```python
from build123d import *

# Parameters (mm, degrees)
SKETCH1_W           = 20
SKETCH1_H           = 5
SKETCH1_R           = 1.5
BOSS_EXTRUDE1_DEPTH = 2


with BuildPart() as part:
    # Sketch1 → Boss-Extrude1 (new body)
    with BuildSketch(Plane(origin=(0, 0, 0), x_dir=(1, 0, 0), z_dir=(0, 1, 0))):
        Rectangle(SKETCH1_W, SKETCH1_H)
        with Locations(Location((-7.5, 0, 0), (0, 0, 270))):
            Circle(SKETCH1_R, mode=Mode.SUBTRACT)
        with Locations(Location((7.5, 0, 0), (0, 0, 270))):
            Circle(SKETCH1_R, mode=Mode.SUBTRACT)
        with Locations(Location((0, 0, 0), (0, 0, 270))):
            Circle(SKETCH1_R, mode=Mode.SUBTRACT)
    extrude(amount=BOSS_EXTRUDE1_DEPTH)


solid = part.part
```
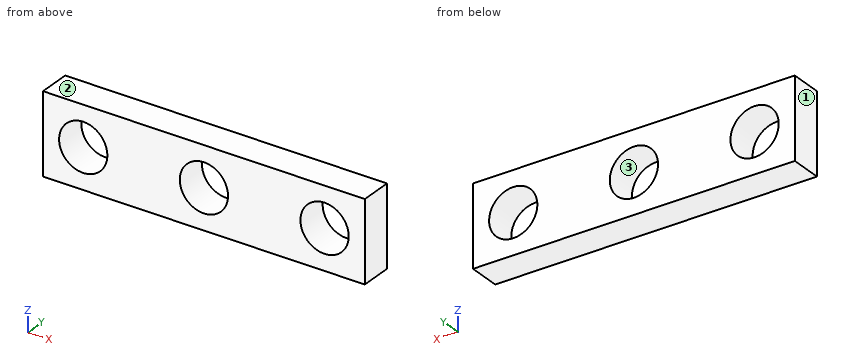
Check sheet for the modelled part. Datum: model origin and axes. Units: mm. Face numbers are marked on the shaded views. Give positions to 0.01 mm unless a question says otherwise; leave off trailing zeros. Write each loop counter-clockwise with the first axis right and the second up, starting at its lowest first coordinate (ties: lowest second). Pieces come first, ordered by that corner, then holes. Notation, with made-up numbers: (33.25, 57.5) -> (52.25, 57.5) arc R21 cw to (52.25, 78.5) -> close; hole circle Ø9 at (55, 42). An arc over 180 degrees is marked (long way). Use CSV: the item, a comma, the result in double quotes. Start each with the question number.
Q1. Scan lines: line 1 along X through (y, z) = (1.2, 0); line 2 along X through (y, z) = (0.6, 1.1); line 3 along Z through (x, y) = (1, 1.45). Record each from-to range of solid material in increasing order.
Q2. Release check for a two-part mould opening along Z. For the marked faces 1, 2 and 3 record: +Z half, -Z half, draft (parallel to the pull), parting line (faces both ways), or undercut.
Q3. Cross-section at D-D on z = -1.2. Enter the section's corners in (x, y).
Q4. Cross-section at B-B on z = 0. Enter the section's corners in (x, y), and give its area (3 significant figures).
Q5. Cross-section at A-A on x = 0. Enter the section's corners in (y, z).
Q6. Depth check by flat-ended pin: P1, Ø1.8, axis at x = 0, z = 0, coming from the -Y side. Enter the tip coordinate at first touch or a pass-through.
Q7. Cross-section at C-C on y = 0.35. Enter the section's corners in (x, z).
Working result:
1,line 1,"x = -10 to -9, -6 to -1.5, 1.5 to 6, 9 to 10"
1,line 2,"x = -10 to -8.52, -6.48 to -1.02, 1.02 to 6.48, 8.52 to 10"
1,line 3,"z = -2.5 to -1.12, 1.12 to 2.5"
2,face 1,"draft"
2,face 2,"+Z half"
2,face 3,"undercut"
3,outline,"(-10, 0) -> (-8.4, 0) -> (-8.4, 2) -> (-10, 2) -> close; (-6.6, 0) -> (-0.9, 0) -> (-0.9, 2) -> (-6.6, 2) -> close; (0.9, 0) -> (6.6, 0) -> (6.6, 2) -> (0.9, 2) -> close; (8.4, 0) -> (10, 0) -> (10, 2) -> (8.4, 2) -> close"
4,outline,"(-10, 0) -> (-9, 0) -> (-9, 2) -> (-10, 2) -> close; (-6, 0) -> (-1.5, 0) -> (-1.5, 2) -> (-6, 2) -> close; (1.5, 0) -> (6, 0) -> (6, 2) -> (1.5, 2) -> close; (9, 0) -> (10, 0) -> (10, 2) -> (9, 2) -> close"
4,area,"22.0 mm^2"
5,outline,"(0, -2.5) -> (2, -2.5) -> (2, -1.5) -> (0, -1.5) -> close; (0, 1.5) -> (2, 1.5) -> (2, 2.5) -> (0, 2.5) -> close"
6,P1,"passes through"
7,outline,"(-10, -2.5) -> (10, -2.5) -> (10, 2.5) -> (-10, 2.5) -> close; hole circle Ø3 at (-7.5, 0); hole circle Ø3 at (0, 0); hole circle Ø3 at (7.5, 0)"
